Input: part model. Units: mm. Frame: model coordinates. A direction names the side the tool comes from. Give positions to 0.01 mm unless a question says otherwise; leave off trailing zeros. Loops run counter-clockwise (first coordinate to the right, second up) from the corner with the lowest first, then second, coordinate; pieces in that order, holes last. Notation, with made-up numbers: M 37.25,51.5 L 47.25,51.5 A17 cw 47.25,83.5 Z; hole C 56,75.5 d10. An arc over 180 degrees is marked long. Answer as a JSON object with one key per item and string values. Group by question number.
1) First-contact query: P1, Ø1, axis at y = 0.5, z = -21, coming from the -X side. Flat tip, straight axial feed; report the tip coordinate or a pass-through.
2) Ray query, L1, parallel to X at y = 2.5, z = -8.89; L2, parallel to Z at x = -42, y = 0.5; L3, parallel to Z at x = -47.5, y = 1.65. Return the intervals inside material, ascending.
3) Section query B-B on x = -2.54. Return loops of the section in (y, z), plus the area to 3 significant figures.
4) Access query for faces 1 (the cylindrical face through (-2.505, 2.216, -46.673)), 2 (the cylindrical face through (-43.87, 2.28, -24.14)), 3 (the cylindrical face through (-6.961, 2.279, -21.124)). Directions: +Z, -Z, +X, -X, +Y, -Y. A direction counts if a zero-diameter tool reaches every point of the face in a straight line with its end or side. Return the directions, or none.
5) Draft query along X for faces 4 (the cylindrical face through (-43.839, 2.279, -39.388)), 5 (the flat face through (-0.952, 2, -54)), 6 (the flat face through (-49, 2, -19.05)). Return one class per face: +X half, -X half, draft (parallel to the pull), parting line (faces both ways), or undercut.
6) Section query C-C on x = -33.5. Count the separate pieces of the cut face and the enclosed holes in it, plus the area to 3 significant figures.
7) Section query A-A on z = -8.89. Return loops of the section in (x, y), plus the area to 3 significant figures.
from build123d import *

# Parameters (mm, degrees)
BOSS_EXTRUDE1_DEPTH     = 4.4958
CUT_EXTRUDE1_DEPTH      = 82.4438593
CUT_EXTRUDE1_DEPTH_BACK = 82.4438593
SKETCH3_R               = 1.5875
CUT_EXTRUDE2_DEPTH      = 82.4438593
CUT_EXTRUDE2_DEPTH_BACK = 82.4438593
SKETCH4_W               = 33.02
SKETCH4_H               = 1.494117647
SKETCH4_H_2             = 1.494117648
FILLET1_R               = 0.762
FILLET2_R               = 2.032
FILLET3_R               = 3.81
FILLET4_R               = 3.81


with BuildPart() as part:
    # Sketch1 → Boss-Extrude1 (new body)
    with BuildSketch(Plane(origin=(0, 0, 0), x_dir=(1, 0, 0), z_dir=(0, 1, 0))):
        Polygon((-50.8, 63.5), (0, 63.5), (0, 44.45), (-6.35, 44.45), (-6.35, 19.05), (0, 19.05), (0, 0), (-50.8, 0), (-50.8, 19.05), (-44.45, 19.05), (-44.45, 44.45), (-50.8, 44.45), align=None)
    extrude(amount=BOSS_EXTRUDE1_DEPTH)

    # Sketch3 → Cut-Extrude1 (cut, two sides: drawn at the far end of the back side and taken through both)
    with BuildSketch(Plane(origin=(0, 4.4958, 0), x_dir=(1, 0, 0), z_dir=(0, 1, 0)).offset(-CUT_EXTRUDE1_DEPTH_BACK)):
        with Locations(Location((-48.26, 8.89, 0), (0, 0, 270))):
            Circle(SKETCH3_R)
        with Locations(Location((-2.54, 8.89, 0), (0, 0, 270))):
            Circle(SKETCH3_R)
        with BuildLine():
            Line((-49.8475, 48.26), (-49.8475, 59.69))
            ThreePointArc((-49.8475, 59.69), (-48.26, 61.2775), (-46.6725, 59.69))
            Line((-46.6725, 59.69), (-46.6725, 48.26))
            ThreePointArc((-46.6725, 48.26), (-48.26, 46.6725), (-49.8475, 48.26))
        make_face()
        with BuildLine():
            Line((-4.1275, 48.26), (-4.1275, 59.69))
            ThreePointArc((-4.1275, 59.69), (-2.54, 61.2775), (-0.9525, 59.69))
            Line((-0.9525, 59.69), (-0.9525, 48.26))
            ThreePointArc((-0.9525, 48.26), (-2.54, 46.6725), (-4.1275, 48.26))
        make_face()
    extrude(amount=CUT_EXTRUDE1_DEPTH + CUT_EXTRUDE1_DEPTH_BACK, mode=Mode.SUBTRACT)

    # Sketch4 → Cut-Extrude2 (cut, two sides: drawn at the far end of the back side and taken through both)
    with BuildSketch(Plane(origin=(0, 4.4958, 0), x_dir=(1, 0, 0), z_dir=(0, 1, 0)).offset(-CUT_EXTRUDE2_DEPTH_BACK)):
        with Locations((-27.94, 34.738235295)):
            Rectangle(SKETCH4_W, SKETCH4_H)
        with Locations((-22.86, 19.797058824)):
            Rectangle(SKETCH4_W, SKETCH4_H)
        with Locations((-27.94, 22.785294118)):
            Rectangle(SKETCH4_W, SKETCH4_H)
        with Locations((-22.86, 25.773529412)):
            Rectangle(SKETCH4_W, SKETCH4_H)
        with Locations((-27.94, 28.761764705)):
            Rectangle(SKETCH4_W, SKETCH4_H)
        with Locations((-22.86, 31.75)):
            Rectangle(SKETCH4_W, SKETCH4_H_2)
        with Locations((-22.86, 37.726470589)):
            Rectangle(SKETCH4_W, SKETCH4_H)
        with Locations((-27.94, 40.714705882)):
            Rectangle(SKETCH4_W, SKETCH4_H)
        with Locations((-22.86, 43.702941177)):
            Rectangle(SKETCH4_W, SKETCH4_H)
    extrude(amount=CUT_EXTRUDE2_DEPTH + CUT_EXTRUDE2_DEPTH_BACK, mode=Mode.SUBTRACT)

    # Fillet1
    # the kernel refuses this fillet: 0.762 mm, written as the material it adds along each edge
    with BuildSketch(Plane(origin=(-39.37, 0, -32.497058824), x_dir=(0, 0, 1), z_dir=(0, 1, 0)), Plane(origin=(-11.43, 0, -29.508823529), x_dir=(-1, 0, 0), z_dir=(0, 1, 0)), Plane(origin=(-11.43, 0, -28.014705882), x_dir=(0, 0, -1), z_dir=(0, 1, 0)), Plane(origin=(-39.37, 0, -31.002941176), x_dir=(1, 0, 0), z_dir=(0, 1, 0)), Plane(origin=(-39.37, 0, -20.544117647), x_dir=(0, 0, 1), z_dir=(0, 1, 0)), Plane(origin=(-39.37, 0, -36.979411765), x_dir=(1, 0, 0), z_dir=(0, 1, 0)), Plane(origin=(-39.37, 0, -42.955882353), x_dir=(1, 0, 0), z_dir=(0, 1, 0)), Plane(origin=(-39.37, 0, -38.473529412), x_dir=(0, 0, 1), z_dir=(0, 1, 0)), Plane(origin=(-39.37, 0, -44.45), x_dir=(0, 0, 1), z_dir=(0, 1, 0)), Plane(origin=(-11.43, 0, -33.991176471), x_dir=(0, 0, -1), z_dir=(0, 1, 0)), Plane(origin=(-11.43, 0, -39.967647059), x_dir=(0, 0, -1), z_dir=(0, 1, 0)), Plane(origin=(-11.43, 0, -35.485294118), x_dir=(-1, 0, 0), z_dir=(0, 1, 0)), Plane(origin=(-11.43, 0, -41.461764706), x_dir=(-1, 0, 0), z_dir=(0, 1, 0))) as fillet1_piece_1:
        with BuildLine():
            CenterArc((FILLET1_R, FILLET1_R), FILLET1_R, 180, 90)
            Line((0, FILLET1_R), (0, 0))
            Line((0, 0), (FILLET1_R, 0))
        make_face()
    extrude(amount=4.4958)
    with BuildSketch(Plane(origin=(-11.43, 4.4958, -22.038235294), x_dir=(0, 0, -1), z_dir=(0, -1, 0)), Plane(origin=(-11.43, 4.4958, -23.532352941), x_dir=(-1, 0, 0), z_dir=(0, -1, 0)), Plane(origin=(-39.37, 4.4958, -25.026470588), x_dir=(1, 0, 0), z_dir=(0, -1, 0)), Plane(origin=(-39.37, 4.4958, -26.520588235), x_dir=(0, 0, 1), z_dir=(0, -1, 0)), Plane(origin=(-39.37, 4.4958, -19.05), x_dir=(1, 0, 0), z_dir=(0, -1, 0))) as fillet1_piece_2:
        with BuildLine():
            CenterArc((FILLET1_R, -FILLET1_R), FILLET1_R, 90, 90)
            Line((0, -FILLET1_R), (0, 0))
            Line((0, 0), (FILLET1_R, 0))
        make_face()
    extrude(amount=4.4958)

    # Fillet2
    fillet2_edges = [part.edges().sort_by_distance(p)[0] for p in [
        (-6.35, 2.2479, -26.520588235),
        (-6.35, 2.2479, -25.026470588),
        (-44.45, 2.2479, -22.038235294),
        (-44.45, 2.2479, -23.532352941),
        (-44.45, 2.2479, -28.014705882),
        (-44.45, 2.2479, -29.508823529),
        (-6.35, 2.2479, -32.497058824),
        (-6.35, 2.2479, -31.002941176),
        (-44.45, 2.2479, -33.991176471),
        (-44.45, 2.2479, -35.485294118),
        (-6.35, 2.2479, -38.473529412),
        (-6.35, 2.2479, -36.979411765),
        (-44.45, 2.2479, -39.967647059),
        (-44.45, 2.2479, -41.461764706),
        (-6.35, 2.2479, -42.955882353),
        (-6.35, 2.2479, -20.544117647),
    ]]
    fillet(fillet2_edges, radius=FILLET2_R)

    # Fillet3
    # the kernel refuses this fillet: 3.81 mm, written as the material it adds along each edge
    with BuildSketch(Plane(origin=(-44.45, 0, -44.45), x_dir=(-1, 0, 0), z_dir=(0, 1, 0))) as fillet3_piece_1:
        with BuildLine():
            CenterArc((3.065547548, 3.81), FILLET3_R, 209.241450743, 60.758549257)
            Line((-0.258939983, 1.948849105), (-0.591388736, 1.762734015))
            ThreePointArc((-0.591388736, 1.762734015), (-0.381, 0.956235294), (-0.381, 0))
            Line((-0.381, 0), (0, -0.381))
            Line((0, -0.381), (3.065547548, -0.381))
            Line((3.065547548, -0.381), (3.065547548, 0))
        make_face()
    extrude(amount=4.4958)

    # Fillet4
    # the kernel refuses this fillet: 3.81 mm, written as the material it adds along each edge
    with BuildSketch(Plane(origin=(-44.45, 0, -19.05), x_dir=(0.1317106342839345, 0, -0.9912882067373362), z_dir=(0, 1, 0))) as fillet4_piece_1:
        with BuildLine():
            CenterArc((3.373042856, 3.540658648), FILLET4_R, 187.568454523, 60.758549257)
            Line((-0.403765212, 3.038841131), (-0.781446019, 2.98865938))
            Line((-0.781446019, 2.98865938), (-0.377680807, -0.050181752))
            Line((-0.377680807, -0.050181752), (0.050181752, -0.377680807))
            ThreePointArc((0.050181752, -0.377680807), (0.998086522, -0.25173445), (1.825269627, -0.354065865))
            Line((1.825269627, -0.354065865), (1.965976284, 0))
        make_face()
    extrude(amount=4.4958)


solid = part.part
Output:
{
 "1": {"P1": "stops at x = -44.52"},
 "2": {"L1": "x = -50.8 to -49.85, -46.67 to -4.13, -0.95 to 0", "L2": "z = -63.5 to -41.46, -39.97 to -35.49, -33.99 to -29.51, -28.01 to -23.53, -22.04 to 0", "L3": "z = -63.5 to -61.08, -46.87 to -44.45, -19.05 to -10.28, -7.5 to 0"},
 "3": {"outline": "M 0,-63.5 L 4.5,-63.5 L 4.5,-61.28 L 0,-61.28 Z; M 0,-46.67 L 4.5,-46.67 L 4.5,-44.45 L 0,-44.45 Z; M 0,-19.05 L 4.5,-19.05 L 4.5,-10.48 L 0,-10.48 Z; M 0,-7.3 L 4.5,-7.3 L 4.5,0 L 0,0 Z", "area": "91.4 mm^2"},
 "4": {"face 1": "+Y, -Y", "face 2": "-X, +Y, -Y", "face 3": "+X, +Y, -Y"},
 "5": {"face 4": "-X half", "face 5": "undercut", "face 6": "draft"},
 "6": {"separate pieces": "10", "enclosed holes": "0", "area": "225 mm^2"},
 "7": {"outline": "M -50.8,0 L -49.85,0 L -49.85,4.5 L -50.8,4.5 Z; M -46.67,0 L -4.13,0 L -4.13,4.5 L -46.67,4.5 Z; M -0.95,0 L 0,0 L 0,4.5 L -0.95,4.5 Z", "area": "200 mm^2"}
}
